Here's how the part is built. I have some questions about the finished solid (model axes, mm). A direction names the side the tool comes from. Give positions to 0.01 mm unless a question says otherwise; leave off trailing zeros. Loops run counter-clockwise (first coordinate to the right, second up) from the corner with the lowest first, then second, coordinate; pieces in that order, holes last. Notation, with made-up numbers: (-12.5, 48) - (43.5, 48) arc R22 cw to (43.5, 63) - close; hole circle Ø7 at (-32.75, 73). An arc over 180 degrees is marked (long way). One line per item, written item: value. Start each with the question number.
```python
from build123d import *

# Parameters (mm, degrees)
SKETCH1_W           = 30
SKETCH1_H           = 30
BOSS_EXTRUDE1_DEPTH = 20
SKETCH2_W           = 20.2
SKETCH2_H           = 20.2
CUT_EXTRUDE1_DEPTH  = 15
SKETCH3_R           = 2.5
CUT_EXTRUDE2_DEPTH  = 40.05124838
SKETCH4_W           = 15
SKETCH4_H           = 15
CUT_EXTRUDE3_DEPTH  = 26.980762114
FILLET2_R           = 5
FILLET1_R           = 0.5
CHAMFER1_SIZE       = 0.2


with BuildPart() as part:
    # Sketch1 → Boss-Extrude1 (new body)
    with BuildSketch(Plane.XY):
        Rectangle(SKETCH1_W, SKETCH1_H)
    extrude(amount=BOSS_EXTRUDE1_DEPTH)

    # Sketch2 → Cut-Extrude1 (cut)
    with BuildSketch(Plane.XY.offset(20)):
        Rectangle(SKETCH2_W, SKETCH2_H)
    extrude(amount=-CUT_EXTRUDE1_DEPTH, mode=Mode.SUBTRACT)

    # Sketch3 → Cut-Extrude2 (cut, through all)
    with BuildSketch(Plane.XZ.offset(15)):
        with Locations(Location((0, 15, 0), (0, 0, 270))):
            Circle(SKETCH3_R)
    extrude(amount=-CUT_EXTRUDE2_DEPTH, mode=Mode.SUBTRACT)

    # Sketch4 → Cut-Extrude3 (cut, through all)
    with BuildSketch(Plane.XY.offset(5)):
        Rectangle(SKETCH4_W, SKETCH4_H)
    extrude(amount=-CUT_EXTRUDE3_DEPTH, mode=Mode.SUBTRACT)

    # Fillet2
    fillet2_edges = [part.edges().sort_by_distance(p)[0] for p in [
        (7.5, 7.5, 2.5),
        (7.5, -7.5, 2.5),
        (-7.5, -7.5, 2.5),
        (-7.5, 7.5, 2.5),
        (15, -15, 10),
        (-15, -15, 10),
        (-15, 15, 10),
        (15, 15, 10),
    ]]
    fillet(fillet2_edges, radius=FILLET2_R)

    # Fillet1
    fillet1_edges = [part.edges().sort_by_distance(p)[0] for p in [
        (10.1, 0, 20),
        (0, 10.1, 20),
        (-10.1, 0, 20),
        (0, -10.1, 20),
        (0, -7.5, 5),
        (0, -7.5, 0),
        (-7.5, 0, 5),
        (-7.5, 0, 0),
        (7.5, 0, 5),
        (7.5, 0, 0),
        (0, 7.5, 5),
        (0, 7.5, 0),
        (0, 15, 0),
        (0, 15, 20),
        (15, 0, 0),
        (0, -15, 0),
        (-15, 0, 0),
        (13.535533906, -13.535533906, 0),
        (-13.535533906, -13.535533906, 0),
        (-13.535533906, 13.535533906, 0),
        (13.535533906, 13.535533906, 0),
        (15, 0, 20),
        (-15, 0, 20),
        (0, -15, 20),
        (13.535533906, -13.535533906, 20),
        (-13.535533906, -13.535533906, 20),
        (-13.535533906, 13.535533906, 20),
        (13.535533906, 13.535533906, 20),
        (-6.035533906, -6.035533906, 5),
        (-6.035533906, -6.035533906, 0),
        (6.035533906, -6.035533906, 5),
        (6.035533906, -6.035533906, 0),
        (6.035533906, 6.035533906, 5),
        (6.035533906, 6.035533906, 0),
        (-6.035533906, 6.035533906, 5),
        (-6.035533906, 6.035533906, 0),
    ]]
    fillet(fillet1_edges, radius=FILLET1_R)

    # Chamfer1
    chamfer1_edges = [part.edges().sort_by_distance(p)[0] for p in [
        (0, 15, 17.5),
        (0, 10.1, 17.5),
        (0, -10.1, 17.5),
        (0, -15, 17.5),
    ]]
    chamfer(chamfer1_edges, length=CHAMFER1_SIZE)


solid = part.part
```
(1) Will this pin go through, and if not, where does the flat tip stop? pin 1 (8 mm diameter, centred on x = 10, y = -7.5, fed in from +Z).
(2) Please list where these lines run through material, in increasing order: probe 1 along X at (y, z) = (-0.75, 10); probe 2 along X at (y, z) = (13.8, 15). Write a range as from..to.
(3) If we section it at B-B on z = 15: List the corners of the cut face in (x, y) for me, plus the area to 3 significant figures.
(4) If we section it at A-A on z = 5.75: List the corners of the cut face in (x, y) for me.
(5) If we section it at C-C on x = 0: Give the number of separate pieces and of enclosed holes in the cut face, plus the area to 3 significant figures.
(6) If we section it at D-D on z = 2.25: List the corners of the cut face in (x, y) for me.
(7) For faces 1 (the face through (15, 0, 10)), 2 (the face through (0, 10.1, 11)), 3 (the face through (6.07, 6, 2.47)), which set-ups out of +Z, -Z, +X, -X, +Y, -Y let a thin tool reach every point of the face, with its end or its side?
(8) If we mould it in two halves opening along Z, with no side actions, what happens to faces 4 (the face through (-7, 7, 0)), 5 (the face through (0.1, -12.6, 17.5)), 6 (the face through (0, 15, 10))? For each: pulls with the +Z half, pulls with the -Z half, needs draft (parallel to the pull), parting line crosses it, or undercut.
Found:
1. pin 1: z = 20
2. probe 1: -15..-10.1, 10.1..15
2. probe 2: -13.25..-2.5, 2.5..13.25
3. outline: (-15, -10) arc R5 ccw to (-10, -15) - (-2.7, -15) - (-2.5, -14.8) - (-2.5, -10.3) - (-2.7, -10.1) - (-10.1, -10.1) - (-10.1, 10.1) - (-2.7, 10.1) - (-2.5, 10.3) - (-2.5, 14.8) - (-2.7, 15) - (-10, 15) arc R5 ccw to (-15, 10) - close; (2.5, -14.8) - (2.7, -15) - (10, -15) arc R5 ccw to (15, -10) - (15, 10) arc R5 ccw to (10, 15) - (2.7, 15) - (2.5, 14.8) - (2.5, 10.3) - (2.7, 10.1) - (10.1, 10.1) - (10.1, -10.1) - (2.7, -10.1) - (2.5, -10.3) - close
3. area: 421 mm^2
4. outline: (-15, -10) arc R5 ccw to (-10, -15) - (10, -15) arc R5 ccw to (15, -10) - (15, 10) arc R5 ccw to (10, 15) - (-10, 15) arc R5 ccw to (-15, 10) - close; hole (-10.1, -10.1) - (10.1, -10.1) - (10.1, 10.1) - (-10.1, 10.1) - close
5. separate pieces: 4
5. enclosed holes: 0
5. area: 172 mm^2
6. outline: (-15, -10) arc R5 ccw to (-10, -15) - (10, -15) arc R5 ccw to (15, -10) - (15, 10) arc R5 ccw to (10, 15) - (-10, 15) arc R5 ccw to (-15, 10) - close; hole (-7.5, -2.5) arc R5 ccw to (-2.5, -7.5) - (2.5, -7.5) arc R5 ccw to (7.5, -2.5) - (7.5, 2.5) arc R5 ccw to (2.5, 7.5) - (-2.5, 7.5) arc R5 ccw to (-7.5, 2.5) - close
7. face 1: +Z, -Z, +X, +Y, -Y
7. face 2: +Z
7. face 3: +Z, -Z
8. face 4: pulls with the -Z half
8. face 5: undercut
8. face 6: needs draft
